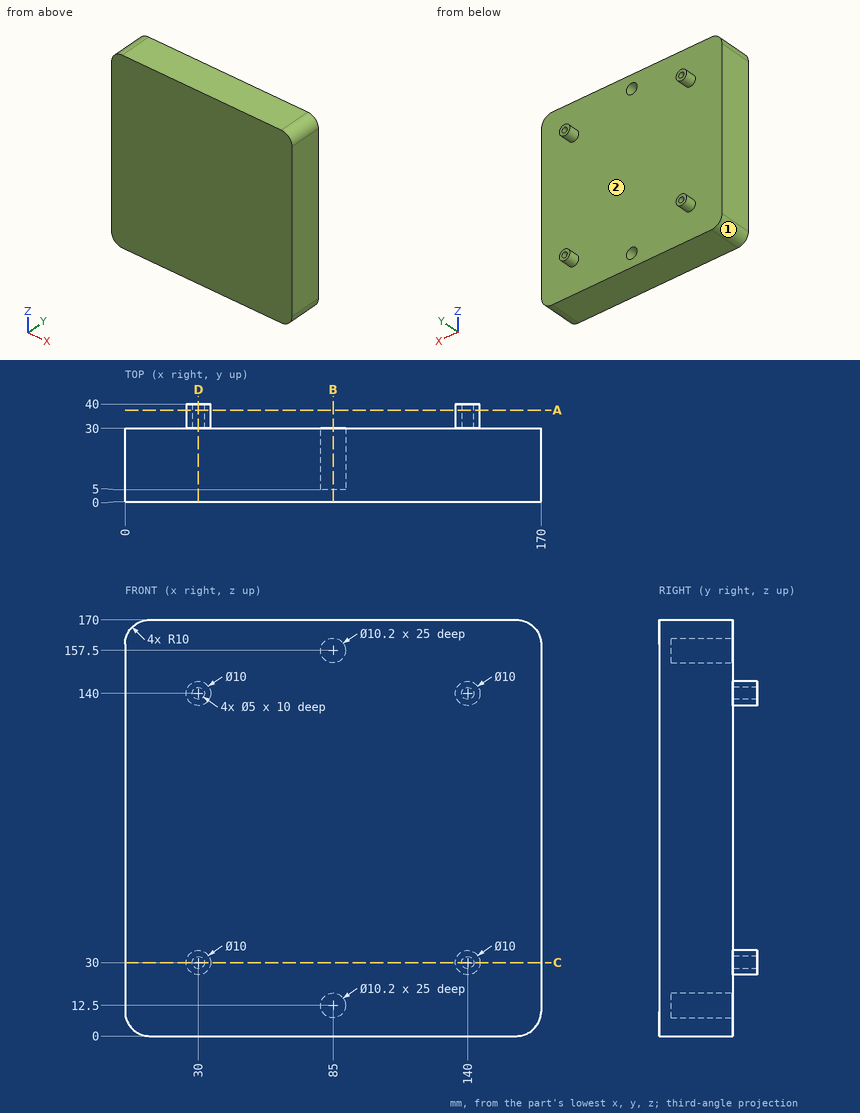
Could you check a few things on this drawing? It's one solid part, dimensions in mm from its lowest x, y, z. A direction names the side the tool comes from. Give positions to 0.01 mm unless a question says otherwise; leave off trailing zeros. Write each loop counter-clockwise with the first axis right and the second up, starting at its lowest first coordinate (ties: lowest second). Pieces come first, ordered by that corner, then holes. Notation, with made-up numbers: (66, 61.5) -> (117, 61.5) arc R28 cw to (117, 88.5) -> close; hole circle Ø6 at (-38.5, -3). An arc over 180 degrees is marked (long way). Write item = value, one per line.
(1) I'm going to push a flat-ended pin straight in: P1, Ø1.5, axis at x = 95, z = 65.5, coming from the +Y side. Where does the tip first touch, or does it pass through?
Worked out:
P1 = 30
(2) I need wall thicknesses on probe 1 along Z at (x, y) = (140, 33.25); probe 2 along Z at (x, y) = (85, 19). Which ranges of each line are inside material? Lowest first, please. Write a range as from..to.
Worked out:
probe_1 = 25..27.5, 32.5..35, 135..137.5, 142.5..145
probe_2 = 0..7.4, 17.6..152.4, 162.6..170
(3) Suppose I cut it at A-A on y = 37.5. Write out the boundary of the cut face in (x, z), then the cut area to 3 significant figures.
Worked out:
outline = circle Ø10 at (30, 30); circle Ø10 at (30, 140); circle Ø10 at (140, 30); circle Ø10 at (140, 140); hole circle Ø5 at (30, 30); hole circle Ø5 at (30, 140); hole circle Ø5 at (140, 30); hole circle Ø5 at (140, 140)
area = 236 mm^2
(4) For the marked faces 1 and 2, which set-ups out of +Z, -Z, +X, -X, +Y, -Y let a thin tool reach every point of the face, with its end or its side?
Worked out:
face_1 = -Z, -X, +Y, -Y
face_2 = +Y
(5) Suppose I cut it at C-C on z = 30. Write out the boundary of the cut face in (x, y).
Worked out:
outline = (0, 0) -> (170, 0) -> (170, 30) -> (145, 30) -> (145, 40) -> (142.5, 40) -> (142.5, 30) -> (137.5, 30) -> (137.5, 40) -> (135, 40) -> (135, 30) -> (35, 30) -> (35, 40) -> (32.5, 40) -> (32.5, 30) -> (27.5, 30) -> (27.5, 40) -> (25, 40) -> (25, 30) -> (0, 30) -> close
(6) Suppose I cut it at D-D on x = 30. Write out the boundary of the cut face in (y, z), then the cut area to 3 significant figures.
Worked out:
outline = (0, 0) -> (30, 0) -> (30, 25) -> (40, 25) -> (40, 27.5) -> (30, 27.5) -> (30, 32.5) -> (40, 32.5) -> (40, 35) -> (30, 35) -> (30, 135) -> (40, 135) -> (40, 137.5) -> (30, 137.5) -> (30, 142.5) -> (40, 142.5) -> (40, 145) -> (30, 145) -> (30, 170) -> (0, 170) -> close
area = 5,200 mm^2
(7) Suppose I cut it at B-B on x = 85. Write out the boundary of the cut face in (y, z), then the cut area to 3 significant figures.
Worked out:
outline = (0, 0) -> (30, 0) -> (30, 7.4) -> (5, 7.4) -> (5, 17.6) -> (30, 17.6) -> (30, 152.4) -> (5, 152.4) -> (5, 162.6) -> (30, 162.6) -> (30, 170) -> (0, 170) -> close
area = 4,590 mm^2
